```python
from build123d import *

# Parameters (mm, degrees)
SKETCH1_W           = 150
SKETCH1_H           = 50
BOSS_EXTRUDE1_DEPTH = 5
SKETCH2_R           = 1.5
CUT_EXTRUDE1_DEPTH  = 10
SKETCH3_R           = 2.5
CUT_EXTRUDE2_DEPTH  = 159.192920196


with BuildPart() as part:
    # Sketch1 → Boss-Extrude1 (new body)
    with BuildSketch(Plane.XY):
        with Locations((75, 25)):
            Rectangle(SKETCH1_W, SKETCH1_H)
    extrude(amount=BOSS_EXTRUDE1_DEPTH)

    # Sketch2 → Cut-Extrude1 (cut)
    with BuildSketch(Plane.XY.offset(5)):
        with Locations((2.5, 5)):
            Circle(SKETCH2_R)
        with Locations((2.5, 47.5)):
            Circle(SKETCH2_R)
        with Locations((147.5, 47.5)):
            Circle(SKETCH2_R)
        with Locations((147.5, 5)):
            Circle(SKETCH2_R)
    extrude(amount=-CUT_EXTRUDE1_DEPTH, mode=Mode.SUBTRACT)

    # Sketch3 → Cut-Extrude2 (cut, through all)
    with BuildSketch(Plane(origin=(0, 0, 0), x_dir=(-1, 0, 0), z_dir=(0, 0, -1))):
        with Locations((-54.86063832, 0.5)):
            Circle(SKETCH3_R)
        with Locations((-47.857694484, 0.5)):
            Circle(SKETCH3_R)
    extrude(amount=-CUT_EXTRUDE2_DEPTH, mode=Mode.SUBTRACT)


solid = part.part
```
Input: part model. Units: mm. Frame: model coordinates. Give positions to 0.01 mm unless a question says otherwise; leave off trailing zeros. Loops run counter-clockwise (first coordinate to the right, second up) from the corner with the lowest first, then second, coordinate; pieces in that order, holes last.
1) Line query: L1, parallel to Y at x = 2.5, z = 2.7; L2, parallel to X at y = 0.5, z = 1.2; L3, parallel to X at y = 6, z = 0.8. Output: solid intervals per line, ascending.
A:
L1: y = 0 to 3.5, 6.5 to 46, 49 to 50
L2: x = 0 to 45.36, 50.36 to 52.36, 57.36 to 150
L3: x = 0 to 1.38, 3.62 to 146.38, 148.62 to 150
2) Mould query, pull axis X, two halves, no side actions, for faces 1 (the cylindrical face through (146, 5, 3)), 2 (the flat face through (0, 25, 2)), 3 (the flat face through (74, 25, 5)). Classes: released by +X, released by -X, zero draft, split by the parting line, or undercut.
A:
face 1: undercut
face 2: released by -X
face 3: zero draft
3) Section query A-A on x = 147.5. Return the cut outline in (y, z).
A:
outline: (0, 0) - (3.5, 0) - (3.5, 5) - (0, 5) - close; (6.5, 0) - (46, 0) - (46, 5) - (6.5, 5) - close; (49, 0) - (50, 0) - (50, 5) - (49, 5) - close
4) Section query B-B on y = 47.5. Return the cut outline in (x, z).
A:
outline: (0, 0) - (1, 0) - (1, 5) - (0, 5) - close; (4, 0) - (146, 0) - (146, 5) - (4, 5) - close; (149, 0) - (150, 0) - (150, 5) - (149, 5) - close
5) Contact query for a flat-ended pin moving along its axis: pin 1 (8 mm diameter, centred on x = 54.86, y = 0.5, fed in from -Z). Output: stop coordinate, or through.
A:
pin 1: stops at z = 0
